Geometry check sheet. Reference: the model listing, model coordinates, mm. A direction names the side the tool comes from. Give positions to 0.01 mm unless a question says otherwise; leave off trailing zeros. Loops run counter-clockwise (first coordinate to the right, second up) from the corner with the lowest first, then second, coordinate; pieces in that order, holes last. Notation, with made-up numbers: (67.5, 62) - (107.5, 62) arc R32 cw to (107.5, 100) - close; hole circle Ø10 at (26, -27). An arc over 180 degrees is marked (long way). One line per question, with ' | ' between items. Start each with the question number.
from build123d import *

# Parameters (mm, degrees)
SKETCH1_R           = 12.5
BOSS_EXTRUDE1_DEPTH = 3
SKETCH2_R           = 1.35
CUT_EXTRUDE1_DEPTH  = 18.930421077
SKETCH4_R           = 2.1
CUT_EXTRUDE2_DEPTH  = 1.5
CIRPATTERN1_COUNT   = 4
SKETCH3_R           = 2.4
BOSS_EXTRUDE2_DEPTH = 8
FILLET1_R           = 1.5


with BuildPart() as part:
    # Sketch1 → Boss-Extrude1 (new body)
    with BuildSketch(Plane(origin=(0, 0, 0), x_dir=(1, 0, 0), z_dir=(0, 1, 0))):
        with Locations(Location((0, 0, 0), (0, 0, 270))):
            Circle(SKETCH1_R)
    extrude(amount=BOSS_EXTRUDE1_DEPTH)

    # Sketch2 → Cut-Extrude1 (cut, through all)
    with BuildSketch(Plane(origin=(0, 3, 0), x_dir=(1, 0, 0), z_dir=(0, 1, 0))):
        with Locations(Location((0, 9.5, 0), (0, 0, 270))):
            Circle(SKETCH2_R)
    cut_extrude1 = extrude(amount=-CUT_EXTRUDE1_DEPTH, mode=Mode.SUBTRACT)

    # Sketch4 → Cut-Extrude2 (cut)
    with BuildSketch(Plane(origin=(0, 3, 0), x_dir=(1, 0, 0), z_dir=(0, 1, 0))):
        with Locations(Location((0, 9.5, 0), (0, 0, 270))):
            Circle(SKETCH4_R)
    cut_extrude2 = extrude(amount=-CUT_EXTRUDE2_DEPTH, mode=Mode.SUBTRACT)

    # CirPattern1: Cut-Extrude1, Cut-Extrude2 ×4 about axis
    cirpattern1_axis = Axis((0, 0, 0), (0, 1, 0))
    add([cut_extrude1.rotate(cirpattern1_axis, i * 360 / CIRPATTERN1_COUNT) for i in range(1, CIRPATTERN1_COUNT)], mode=Mode.SUBTRACT)
    add([cut_extrude2.rotate(cirpattern1_axis, i * 360 / CIRPATTERN1_COUNT) for i in range(1, CIRPATTERN1_COUNT)], mode=Mode.SUBTRACT)

    # Sketch3 → Boss-Extrude2 (add)
    with BuildSketch(Plane(origin=(0, 3, 0), x_dir=(1, 0, 0), z_dir=(0, 1, 0))):
        with Locations(Location((0, 0, 0), (0, 0, 270))):
            Circle(SKETCH3_R)
    extrude(amount=BOSS_EXTRUDE2_DEPTH)

    # Fillet1
    # the kernel refuses this fillet: 1.5 mm, written as the material it adds along each edge
    with BuildSketch(Plane(origin=(0, 3, 0), x_dir=(0, 0, 1), z_dir=(-1, 0, 0))) as fillet1_piece_1:
        with BuildLine():
            CenterArc((2.4 + FILLET1_R, FILLET1_R), FILLET1_R, 180, 90)
            Line((2.4, FILLET1_R), (2.4, 0))
            Line((2.4, 0), (2.4 + FILLET1_R, 0))
        make_face()
    revolve(axis=Axis((0, 3, 0), (0, 1, 0)))
    # the kernel refuses this fillet: 1.5 mm, written as the material it takes off along each edge
    with BuildSketch(Plane(origin=(0, 3, 0), x_dir=(0, 0, 1), z_dir=(-1, 0, 0))) as fillet1_2_piece_1:
        with BuildLine():
            CenterArc((12.5 - FILLET1_R, -FILLET1_R), FILLET1_R, 0, 90)
            Line((12.5 - FILLET1_R, 0), (12.5, 0))
            Line((12.5, 0), (12.5, -FILLET1_R))
        make_face()
    revolve(axis=Axis((0, 3, 0), (0, 1, 0)), mode=Mode.SUBTRACT)


solid = part.part
(1) Tool access check on faces 1 (the face through (-8.212, 0.76, -0.406)), 2 (the face through (0, 1.5, -8)). Record the directions out of +Z, -Z, +X, -X, +Y, -Y that give a thin tool (end or side, any length) a straight path to the whole face; none if there is none.
(2) Section check A-A, the plane z = 0. Record the boundary of the cut face in (x, y), and give its area (3 significant figures).
(3) Material ranges on line 1 (Z direction, x = 0.25, y = 2.5); line 2 (Y direction, x = -7.25, z = -1.25); line 3 (X direction, y = 2.1, z = -9.5), recorded low to high.
(4) Section check B-B, the plane y = 3.5. Record the boundary of the cut face in (x, z), and give its area (3 significant figures).
(5) Mould release check, pull along X, two halves, no side actions. Record for faces 3 (the face through (2.024, 7.704, 1.29)), 4 (the face through (0, 3, 5)), 5 (the face through (7.497, 2.26, 0.631)): pulls with the +X half, pulls with the -X half, needs draft (parallel to the pull), parting line crosses it, or undercut.
(6) Depth check by flat-ended pin: pin 1 Ø10 at (x, z) = (6.5, -5) entering from -Y; pin 2 Ø3 at (x, z) = (9.5, 0) entering from +Y; pin 3 Ø4 at (x, y) = (9, 4) entering from +Z; pin 4 Ø3 at (y, z) = (7, -1) entering from +X. Enter the tip coordinate at first touch or a pass-through.
Numbers:
1) face 1: +Y, -Y | face 2: +Y
2) outline: (-12.5, 0) - (-10.85, 0) - (-10.85, 1.5) - (-11.6, 1.5) - (-11.6, 2.87) arc R1.5 ccw to (-12.5, 1.5) - close; (-8.15, 0) - (8.15, 0) - (8.15, 1.5) - (7.4, 1.5) - (7.4, 3) - (3.9, 3) arc R1.5 cw to (2.4, 4.5) - (2.4, 11) - (-2.4, 11) - (-2.4, 4.5) arc R1.5 cw to (-3.9, 3) - (-7.4, 3) - (-7.4, 1.5) - (-8.15, 1.5) - close; (10.85, 0) - (12.5, 0) - (12.5, 1.5) arc R1.5 ccw to (11.6, 2.87) - (11.6, 1.5) - (10.85, 1.5) - close | area: 92.7 mm^2
3) line 1: -12.12 to -11.59, -7.41 to 7.41, 11.59 to 12.12 | line 2: 0 to 3 | line 3: -7.93 to -2.1, 2.1 to 7.93
4) outline: circle Ø5.56 at (0, 0) | area: 24.3 mm^2
5) face 3: parting line crosses it | face 4: needs draft | face 5: undercut
6) pin 1: y = 0 | pin 2: y = 1.5 | pin 3: z = 9.38 | pin 4: x = 2.4
